Source: CAD feature listing. Evaluate the final solid. Frame: model axes, mm. Face numbers are marked on the shaded views. A direction names the side the tool comes from. Coordinates: 2 decimals unless noted, no trailing zeros. Write each loop counter-clockwise with the first axis right and the second up, starting at its lowest first coordinate (ties: lowest second). Pieces come first, ordered by that corner, then holes. Notation, with made-up numbers: M 22.25,78 L 49.25,78 A18 ccw 49.25,89 Z; hole C 64,82.5 d2. An arc over 180 degrees is marked long. Answer as CSV lines item,"result". Start each with the question number.
1. Reachability of the marked faces 1, 2, 3 and 4 from +Z, -Z, +X, -X, +Y, -Y: full face, straight path, thin tool, end or side. Return the list, or none.
2. Section C-C on z = 26. Return the cut outline in (x, y), plus the area to 3 significant figures.
3. Contact query for flat-ended pins moving along their axis: pin 1 Ø5 at (x, z) = (40.5, 7) entering from +Y; pin 2 Ø21 at (x, y) = (78.5, -42) entering from +Z; pin 3 Ø0.8 at (y, z) = (55.5, 16) entering from -X. Output: stop coordinate, or through.
4. Line query: probe 1 along X at (y, z) = (-13, 6.15); probe 2 along Y at (x, z) = (81, 22); probe 3 along Y at (x, z) = (-44, 29). Output: solid intervals per line, ascending. Write a range as [from, to].
5. Section D-D on y = 13. Return the cut outline in (x, z), plus the area to 3 significant figures.
6. Section A-A on y = 0. Return the cut outline in (x, z), plus the area to 3 significant figures.
7. Section B-B on x = -21.5. Return the cut outline in (y, z).
```python
from build123d import *

# Parameters (mm, degrees)
F0_W      = 127
F0_H      = 99
F2_DEPTH  = 6.5
F0_W_2    = 118
F0_H_2    = 89
F3_DEPTH  = 0.5
F5_DEPTH  = 25
F1_R      = 5.25
F6_DEPTH  = 6.5
F7_W      = 6
F7_H      = 19
F7_W_2    = 17
F7_R      = 5.25
F8_DEPTH  = 5.5
F9_R      = 5.25
F10_DEPTH = 5
F11_W     = 1
F11_H     = 16
F12_DEPTH = 1


with BuildPart() as f2:
    # F0 (on Top) → F2 (new body)
    with BuildSketch(Plane.XY):
        Polygon((97, 56), (65, 56), (65, 54.5), (-64, 54.5), (-64, -54.5), (65, -54.5), (65, -56), (97, -56), align=None)
        with Locations((1.5, 2)):
            Rectangle(F0_W, F0_H, mode=Mode.SUBTRACT)
    extrude(amount=F2_DEPTH)

    # F0 (on Top) → F3 (join)
    with BuildSketch(Plane.XY):
        with Locations((1.5, 2)):
            Rectangle(F0_W, F0_H)
        Rectangle(F0_W_2, F0_H_2, mode=Mode.SUBTRACT)
    extrude(amount=F3_DEPTH)

    # F4 (on face) → F5 (join)
    with BuildSketch(Plane.XY.offset(6.5)):
        Polygon((97, -56), (97, 56), (65, 56), (65, 54.5), (-64, 54.5), (-64, -54.5), (65, -54.5), (65, -56), align=None)
        Polygon((-63, -53.5), (-63, 53.5), (66, 53.5), (66, 55), (96, 55), (96, -55), (66, -55), (66, -53.5), align=None, mode=Mode.SUBTRACT)
    extrude(amount=F5_DEPTH)

    # F1 (on face) → F6 (cut, through all)
    with BuildSketch(Plane.XY):
        with Locations((83.5, -42.25)):
            Circle(F1_R)
        with Locations((83.5, 42.25)):
            Circle(F1_R)
        with Locations((85, -26)):
            Circle(F1_R)
        with Locations((85, -13)):
            Circle(F1_R)
        with Locations((85, 0)):
            Circle(F1_R)
        with Locations((85, 13)):
            Circle(F1_R)
        with Locations((85, 26)):
            Circle(F1_R)
    extrude(amount=F6_DEPTH, mode=Mode.SUBTRACT)

    # F7 (on face) → F8 (cut)
    with BuildSketch(Plane.XY.offset(6.5)):
        with Locations((72, 42.25)):
            Rectangle(F7_W, F7_H)
        with Locations((83.5, 42.25)):
            Rectangle(F7_W_2, F7_H)
        with Locations((83.5, 42.25)):
            Circle(F7_R, mode=Mode.SUBTRACT)
        with Locations((72, -42.25)):
            Rectangle(F7_W, F7_H)
        with Locations((83.5, -42.25)):
            Rectangle(F7_W_2, F7_H)
        with Locations((83.5, -42.25)):
            Circle(F7_R, mode=Mode.SUBTRACT)
    extrude(amount=-F8_DEPTH, mode=Mode.SUBTRACT)

    # F9 (on face) → F10 (cut)
    with BuildSketch(Plane.XY):
        with BuildLine():
            Line((97, -31.5), (97, 31.5))
            Line((97, 31.5), (78, 31.5))
            ThreePointArc((78, 31.5), (74.464466, 30.035534), (73, 26.5))
            Line((73, 26.5), (73, -26.5))
            ThreePointArc((73, -26.5), (74.464466, -30.035534), (78, -31.5))
            Line((78, -31.5), (97, -31.5))
        make_face()
        with Locations((85, 0)):
            Circle(F9_R, mode=Mode.SUBTRACT)
    extrude(amount=F10_DEPTH, mode=Mode.SUBTRACT)

    # F11 (on face) → F12 (cut)
    with BuildSketch(Plane.XY.offset(31.5)):
        with Locations((-63.5, -2)):
            Rectangle(F11_W, F11_H)
    extrude(amount=-F12_DEPTH, mode=Mode.SUBTRACT)


solid = f2.part
```
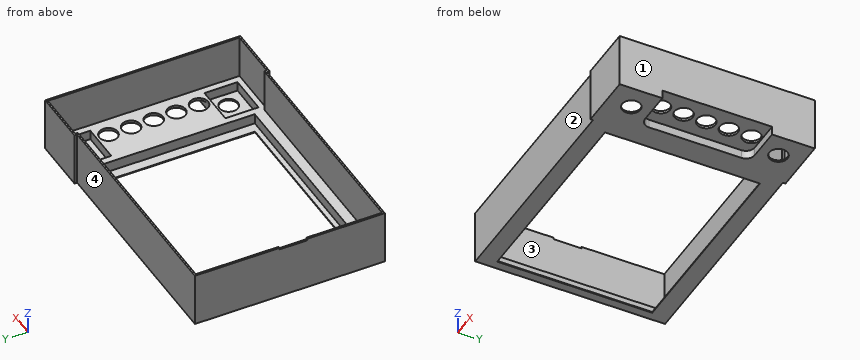
Values:
1,face 1,"+Z, -Z, +X, +Y, -Y"
1,face 2,"+Z, -Z, -X, -Y"
1,face 3,"+Z"
1,face 4,"+Z, -Z, -X, +Y"
2,outline,"M -64,-54.5 L 65,-54.5 L 65,-56 L 97,-56 L 97,56 L 65,56 L 65,54.5 L -64,54.5 Z; hole M -63,-53.5 L 66,-53.5 L 66,-55 L 96,-55 L 96,55 L 66,55 L 66,53.5 L -63,53.5 Z"
2,area,"542 mm²"
3,pin 1,"y = 54.5"
3,pin 2,"z = 6.5"
3,pin 3,"x = 65"
4,probe 1,"[-64, -62], [65, 79.75], [90.25, 97]"
4,probe 2,"[-56, -55], [55, 56]"
4,probe 3,"[-54.5, -53.5], [53.5, 54.5]"
5,outline,"M -64,0 L -59,0 L -59,0.5 L -62,0.5 L -62,6.5 L -63,6.5 L -63,31.5 L -64,31.5 Z; M 59,0 L 73,0 L 73,5 L 79.75,5 L 79.75,6.5 L 65,6.5 L 65,0.5 L 59,0.5 Z; M 90.25,5 L 97,5 L 97,31.5 L 96,31.5 L 96,6.5 L 90.25,6.5 Z"
5,area,"140 mm²"
6,outline,"M -64,0 L -59,0 L -59,0.5 L -62,0.5 L -62,6.5 L -63,6.5 L -63,30.5 L -64,30.5 Z; M 59,0 L 73,0 L 73,5 L 79.75,5 L 79.75,6.5 L 65,6.5 L 65,0.5 L 59,0.5 Z; M 90.25,5 L 97,5 L 97,31.5 L 96,31.5 L 96,6.5 L 90.25,6.5 Z"
6,area,"139 mm²"
7,outline,"M -54.5,0 L -44.5,0 L -44.5,0.5 L -47.5,0.5 L -47.5,6.5 L -53.5,6.5 L -53.5,31.5 L -54.5,31.5 Z; M 44.5,0 L 54.5,0 L 54.5,31.5 L 53.5,31.5 L 53.5,6.5 L 51.5,6.5 L 51.5,0.5 L 44.5,0.5 Z"
